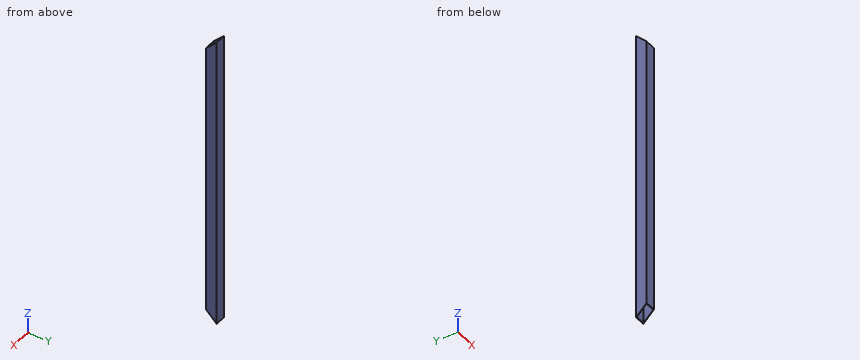
```python
from build123d import *

# Parameters (mm, degrees)
SKETCH1_W           = 50
SKETCH1_H           = 50
SKETCH1_W_2         = 46
SKETCH1_H_2         = 46
BOSS_EXTRUDE1_DEPTH = 1414.3
CUT_EXTRUDE1_DEPTH  = 1416.404355652


with BuildPart() as part:
    # Sketch1 → Boss-Extrude1 (new body)
    with BuildSketch(Plane.XY):
        Rectangle(SKETCH1_W, SKETCH1_H)
        Rectangle(SKETCH1_W_2, SKETCH1_H_2, mode=Mode.SUBTRACT)
    extrude(amount=BOSS_EXTRUDE1_DEPTH)

    # Sketch2 → Cut-Extrude1 (cut, through all)
    with BuildSketch(Plane(origin=(25, 0, 0), x_dir=(0, 0, -1), z_dir=(1, 0, 0))):
        Polygon((-1414.3, 25), (-1414.3, -25), (-1364.3, -25), align=None)
        Polygon((0, 25), (0, -25), (-50, -25), align=None)
    extrude(amount=-CUT_EXTRUDE1_DEPTH, mode=Mode.SUBTRACT)


solid = part.part
```
Can you work these out from the model? Positions are in its coordinate system, mm. Give positions to 0.01 mm unless a question says otherwise; leave off trailing zeros. Order: outer loops, then holes, each group sorted by start corner. A loop starts at its lowest first (then second) coordinate and runs counter-clockwise, first axis right, second up. Notation, with made-up numbers: M 16.25,79.25 L 24.25,79.25 A16 ccw 24.25,105.25 Z; hole C 2,-4 d2. An arc over 180 degrees is marked long. One line per item, written item: value.
1) I want a section at A-A, the plane y = -14. List the corners of the cut face in (x, z) for me, plus the area to 3 significant figures.
Answer sheet:
outline: M -25,39 L -23,39 L -23,1375.3 L -25,1375.3 Z; M 23,39 L 25,39 L 25,1375.3 L 23,1375.3 Z
area: 5,350 mm^2
2) I want a section at B-B, the plane x = 8. List the corners of the cut face in (y, z) for me, plus the area to 3 significant figures.
Answer sheet:
outline: M -25,50 L -23,48 L -23,1366.3 L -25,1364.3 Z; M 23,2 L 25,0 L 25,1414.3 L 23,1412.3 Z
area: 5,460 mm^2
3) I want a section at C-C, the plane z = 795. List the corners of the cut face in (x, y) for me, plus the area to 3 significant figures.
Answer sheet:
outline: M -25,-25 L 25,-25 L 25,25 L -25,25 Z; hole M -23,-23 L 23,-23 L 23,23 L -23,23 Z
area: 384 mm^2
4) Please list where this line runs through material, in increasing order: line 1 along X through (y, z) = (7.5, 822.5).
Answer sheet:
line 1: x = -25 to -23, 23 to 25
